```python
from build123d import *

# Parameters (mm, degrees)
EXTRUDE_THIN1_DEPTH = 333.375
FILLET1_R           = 1.27


with BuildPart() as part:
    # Sketch1 → Extrude-Thin1 (new body)
    with BuildSketch(Plane.XY):
        with BuildLine():
            Line((0, 15.160625), (-1.5875, 15.160625))
            ThreePointArc((-1.5875, 15.160625), (-8.061044421, 14.097490008), (-13.854545455, 11.019766961))
            ThreePointArc((-13.854545455, 11.019766961), (-19.30725231, 8.123086446), (-25.4, 7.122488807))
            Line((-25.4, 7.122488807), (-26.9875, 7.122488807))
            Line((-26.9875, 7.122488807), (-26.9875, 3.175))
            Line((-26.9875, 3.175), (-33.3375, 3.175))
            Line((-33.3375, 3.175), (-33.3375, 0))
            Line((-33.3375, 0), (-17.4625, 0))
            Line((-17.4625, 0), (-17.4625, 1.27))
            Line((-17.4625, 1.27), (-32.0675, 1.27))
            Line((-32.0675, 1.27), (-32.0675, 1.905))
            Line((-32.0675, 1.905), (-25.7175, 1.905))
            Line((-25.7175, 1.905), (-25.7175, 5.852488807))
            Line((-25.7175, 5.852488807), (-25.4, 5.852488807))
            ThreePointArc((-25.4, 5.852488807), (-18.90106913, 6.919792956), (-13.084848485, 10.009585505))
            ThreePointArc((-13.084848485, 10.009585505), (-7.654861242, 12.894196518), (-1.5875, 13.890625))
            Line((-1.5875, 13.890625), (0, 13.890625))
            Line((0, 13.890625), (0, 15.160625))
        make_face()
    extrude(amount=-EXTRUDE_THIN1_DEPTH)

    # Fillet1
    fillet1_edges = [part.edges().sort_by_distance(p)[0] for p in [
        (-33.3375, 0, -166.6875),
        (-33.3375, 3.175, -166.6875),
        (-26.9875, 7.122488807, -166.6875),
        (-25.7175, 1.905, -166.6875),
    ]]
    fillet(fillet1_edges, radius=FILLET1_R)


solid = part.part
```
Part model, mm, in its own coordinate system. A direction names the side the tool comes from. Round coordinates to 2 decimals unless told otherwise and drop trailing zeros. Write each loop counter-clockwise with the first axis right and the second up, starting at its lowest first coordinate (ties: lowest second). Pieces come first, ordered by that corner, then holes.
Item 1: Drop flat-ended pins along their axis: pin 1 Ø4.5 at (x, z) = (-26, -215.5) entering from +Y; pin 2 Ø10 at (x, z) = (-15.5, -224) entering from +Y; pin 3 Ø1.7 at (x, z) = (-0.5, -167) entering from -Y. Give the stop position or say it passes through.
Results:
pin 1: stops at y = 7.19
pin 2: stops at y = 13.09
pin 3: stops at y = 13.89
Item 2: Cut at A-A, the plane x = -21.5. Give the cut face in (y, z) (3 decimals), plus the area to 3 significant figures.
Results:
outline: (0, -333.375) - (1.27, -333.375) - (1.27, 0) - (0, 0) - close; (6.23, -333.375) - (7.526, -333.375) - (7.526, 0) - (6.23, 0) - close
area: 855 mm2
Item 3: Which spindle directions (+Z, -Z, +X, -X, +Y, -Y) get a long thin tool onto all of the face, cutting with end or side? Do faces 5 (the flat face through (-30, 1.905, -164)), 6 (the flat face through (-25, 0, -164)). Say none if no direction does.
Results:
face 5: +Z, -Z, +X
face 6: +Z, -Z, +X, -X, -Y
Item 4: Two-plate mould, pull along Y, no slides. Class faces 1 (the flat face through (-29, 3.175, -164)), 2 (the flat face through (-20, 7, -333.375)), 3 (the flat face through (-25, 1.27, -164)), 4 (the cylindrical face through (-18.99, 6.89, -164.35)): +Y half, -Y half, draft (parallel to the pull), parting line (faces both ways), or undercut.
Results:
face 1: +Y half
face 2: draft
face 3: undercut
face 4: undercut
Item 5: Probe L1, parallel to Y at x = -32, z = -160 (3 decimals); L2, parallel to Y at x = -2, z = -261.5; L3, parallel to Y at x = -2.5, z = -93. List the from-to ranges inside material, lowest first.
Results:
L1: y = 0 to 1.27, 1.905 to 3.175
L2: y = 13.89 to 15.16
L3: y = 13.87 to 15.14
